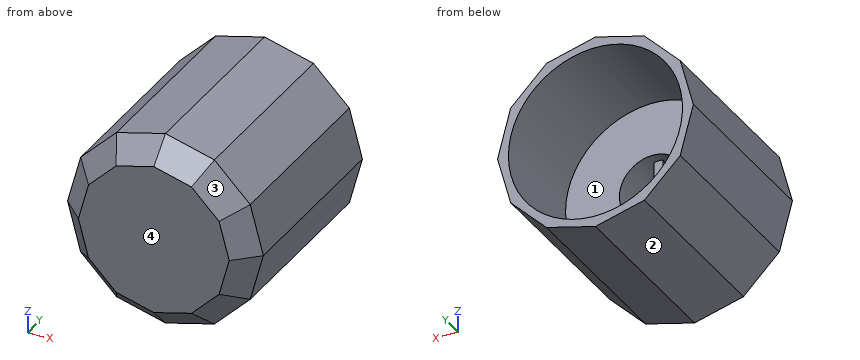
from build123d import *

# Parameters (mm, degrees)
BOSS_EXTRUDE1_DEPTH = 19
SKETCH2_R           = 8
CUT_EXTRUDE1_DEPTH  = 9.8
SKETCH3_R           = 3.05
CUT_EXTRUDE2_DEPTH  = 14
CHAMFER1_SIZE       = 2
SKETCH4_R           = 3.3
BOSS_EXTRUDE2_DEPTH = 3.2
BOSS_EXTRUDE3_DEPTH = 4
SKETCH7_R           = 3.05
BOSS_EXTRUDE4_DEPTH = 1
SKETCH8_R           = 3.05
BOSS_EXTRUDE5_DEPTH = 2


with BuildPart() as part:
    # Sketch1 → Boss-Extrude1 (new body)
    with BuildSketch(Plane(origin=(0, 0, 0), x_dir=(1, 0, 0), z_dir=(0, 1, 0))):
        Polygon((0, 9), (-4.5, 7.794228634), (-7.794228634, 4.5), (-9, 0), (-7.794228634, -4.5), (-4.5, -7.794228634), (0, -9), (4.5, -7.794228634), (7.794228634, -4.5), (9, 0), (7.794228634, 4.5), (4.5, 7.794228634), align=None)
    extrude(amount=BOSS_EXTRUDE1_DEPTH)

    # Sketch2 → Cut-Extrude1 (cut)
    with BuildSketch(Plane(origin=(0, 19, 0), x_dir=(1, 0, 0), z_dir=(0, 1, 0))):
        Circle(SKETCH2_R)
    extrude(amount=-CUT_EXTRUDE1_DEPTH, mode=Mode.SUBTRACT)

    # Sketch3 → Cut-Extrude2 (cut)
    with BuildSketch(Plane(origin=(0, 9.2, 0), x_dir=(1, 0, 0), z_dir=(0, 1, 0))):
        Circle(SKETCH3_R)
    extrude(amount=-CUT_EXTRUDE2_DEPTH, mode=Mode.SUBTRACT)

    # Chamfer1
    chamfer1_edges = [part.edges().sort_by_distance(p)[0] for p in [
        (6.147114317, 0, -6.147114317),
        (8.397114317, 0, -2.25),
        (8.397114317, 0, 2.25),
        (6.147114317, 0, 6.147114317),
        (2.25, 0, 8.397114317),
        (-2.25, 0, 8.397114317),
        (-6.147114317, 0, 6.147114317),
        (-8.397114317, 0, 2.25),
        (-8.397114317, 0, -2.25),
        (-6.147114317, 0, -6.147114317),
        (-2.25, 0, -8.397114317),
        (2.25, 0, -8.397114317),
    ]]
    chamfer(chamfer1_edges, length=CHAMFER1_SIZE)

    # Sketch4 → Boss-Extrude2 (add)
    with BuildSketch(Plane(origin=(0, 1, 0), x_dir=(1, 0, 0), z_dir=(0, 1, 0))):
        Circle(SKETCH4_R)
    extrude(amount=BOSS_EXTRUDE2_DEPTH)

    # Sketch6 → Boss-Extrude3 (add)
    with BuildSketch(Plane(origin=(0, 4.2, 0), x_dir=(1, 0, 0), z_dir=(0, 1, 0))):
        Polygon((-0.4, 0), (-0.4, 3.838549479), (0.4, 3.838549479), (0.4, -4.35363468), (-0.4, -4.35363468), align=None)
    extrude(amount=BOSS_EXTRUDE3_DEPTH)

    # Sketch7 → Boss-Extrude4 (add)
    with BuildSketch(Plane(origin=(0, 1, 0), x_dir=(-1, 0, 0), z_dir=(0, -1, 0))):
        Circle(SKETCH7_R)
    extrude(amount=BOSS_EXTRUDE4_DEPTH)

    # Sketch8 → Boss-Extrude5 (add)
    with BuildSketch(Plane(origin=(0, 4.2, 0), x_dir=(1, 0, 0), z_dir=(0, 1, 0))):
        Circle(SKETCH8_R)
    extrude(amount=BOSS_EXTRUDE5_DEPTH)


solid = part.part
Work out the finished part from the listing and answer in its coordinate system (mm). Face numbers are marked on the shaded views. Round coordinates to 2 decimals unless told otherwise and drop trailing zeros. Order: outer loops, then holes, each group sorted by start corner. A loop starts at its lowest first (then second) coordinate and runs counter-clockwise, first axis right, second up. Notation, with made-up numbers: M 34,76 L 67,76 A12 ccw 67,97 Z; hole C 0.5,42 d9. An arc over 180 degrees is marked long. One line per item, written item: value.
Q1. Find section B-B on y = 3.75. Write down the section's boundary in (x, z), then the cut area to 3 significant figures.
Derived:
outline: M -9,0 L -7.79,-4.5 L -4.5,-7.79 L 0,-9 L 4.5,-7.79 L 7.79,-4.5 L 9,0 L 7.79,4.5 L 4.5,7.79 L 0,9 L -4.5,7.79 L -7.79,4.5 Z
area: 243 mm²
Q2. Find section C-C on x = -5. Write down the section's boundary in (y, z) (3 decimals), then the cut area to 3 significant figures.
Derived:
outline: M 0,-4.466 L 2,-7.294 L 19,-7.294 L 19,-6.245 L 9.2,-6.245 L 9.2,6.245 L 19,6.245 L 19,7.294 L 2,7.294 L 0,4.466 Z
area: 149 mm²
Q3. Determine the mould class of the marked faces 1, 2, 3 and 4 for opening direction X: released by +X, released by -X, zero draft, split by the parting line, or undercut.
Derived:
face 1: undercut
face 2: released by -X
face 3: released by +X
face 4: zero draft
Q4. Find section A-A on y = 11.5. Write down the section's boundary in (x, z), then the cut area to 3 significant figures.
Derived:
outline: M -9,0 L -7.79,-4.5 L -4.5,-7.79 L 0,-9 L 4.5,-7.79 L 7.79,-4.5 L 9,0 L 7.79,4.5 L 4.5,7.79 L 0,9 L -4.5,7.79 L -7.79,4.5 Z; hole C 0,0 d16
area: 41.9 mm²
Q5. Flat-ended cylindrical pins translate along their axes: pin 1 (0.6 mm diameter, centred on y = 7.5, z = 1, fed in from +X); pin 2 (2 mm diameter, centred on x = 5, z = 3.5, fed in from +Y); pin 3 (0.9 mm diameter, centred on x = 0, z = -1, fed in from +Y). Find the tip coordinate at first contact, or state that the pin passes through.
Derived:
pin 1: x = 8.81
pin 2: y = 9.2
pin 3: y = 8.2
Q6. Straight lines are drawn through the part: line 1 (X direction, y = 7.05, z = 0); line 2 (Z direction, x = 0, y = 17); line 3 (Z direction, x = 4.5, y = 4.5). For each, find the intervals that lie inside material, in ascending order.
Derived:
line 1: -9 to -3.05, -0.4 to 0.4, 3.05 to 9
line 2: -9 to -8, 8 to 9
line 3: -7.79 to 7.79
Q7. Find section D-D on z = -0.5. Write down the section's boundary in (x, y), then the cut area to 3 significant figures.
Derived:
outline: M -8.87,2 L -6.8,0 L 6.8,0 L 8.87,2 L 8.87,19 L 7.98,19 L 7.98,9.2 L 3.01,9.2 L 3.01,6.2 L 0.4,6.2 L 0.4,8.2 L -0.4,8.2 L -0.4,6.2 L -3.01,6.2 L -3.01,9.2 L -7.98,9.2 L -7.98,19 L -8.87,19 Z
area: 160 mm²
